For this review, take the finished solid that the model builds, in its own axes (mm). A direction names the side the tool comes from. Give positions to 0.01 mm unless a question says otherwise; leave off trailing zeros. Loops run counter-clockwise (first coordinate to the right, second up) from the corner with the lowest first, then second, coordinate; pieces in that order, holes last. Notation, with made-up numbers: (-11.5, -21.5) - (37.5, -21.5) arc R15 cw to (37.5, -8.5) - close; hole circle Ø9 at (2.5, 4). An arc over 180 degrees is marked (long way). Answer as CSV lines item,"result".
from build123d import *

# Parameters (mm, degrees)
F0_W     = 38.1
F0_H     = 12.7
F1_DEPTH = 25.4
F3_DEPTH = 12.7


with BuildPart() as f1:
    # F0 (on Front) → F1 (new body)
    with BuildSketch(Plane.XZ):
        with Locations((19.05, 6.35)):
            Rectangle(F0_W, F0_H)
    extrude(amount=F1_DEPTH)

    # F2 (on Front) → F3 (join)
    with BuildSketch(Plane.XZ):
        Polygon((0, 31.995658), (0, 12.945658), (0, 0), (38.1, 0), (38.1, 31.995658), (25.4, 31.995658), (25.4, 25.645658), (12.7, 25.645658), (12.7, 31.995658), align=None)
    extrude(amount=F3_DEPTH)


solid = f1.part
1) Consider section B-B on y = -7.75. Write out the cut boundary in (x, z).
From the geometry:
outline,"(0, 0) - (38.1, 0) - (38.1, 32) - (25.4, 32) - (25.4, 25.65) - (12.7, 25.65) - (12.7, 32) - (0, 32) - close"
2) Wall thickness on line 1 (Z direction, x = 16.5, y = -9.25); line 2 (Z direction, x = 20.5, y = -23); line 3 (Y direction, x = 24, z = 21.5): over which ranges is each line inside the solid? List them lowest first. Write a range as from..to.
From the geometry:
line 1,"z = 0..25.65"
line 2,"z = 0..12.7"
line 3,"y = -12.7..0"
3) Insertion check: P1, Ø14, axis at x = 26, y = -20, coming from the +Z side; P2, Ø4, axis at x = 16, y = -8.5, coming from the +Z side; P3, Ø5, axis at x = 18, z = 22.5, coming from the -Y side. Each pin has a flat end and moves straight along its axis. Give the tip position at first contact, or say it passes through.
From the geometry:
P1,"stops at z = 12.7"
P2,"stops at z = 25.65"
P3,"stops at y = -12.7"
4) Consider section C-C on x = 7. Write out the cut boundary in (y, z).
From the geometry:
outline,"(-25.4, 0) - (0, 0) - (0, 32) - (-12.7, 32) - (-12.7, 12.7) - (-25.4, 12.7) - close"
5) Consider section D-D on z = 14. Write out the cut boundary in (x, y), and give its area (3 significant figures).
From the geometry:
outline,"(0, -12.7) - (38.1, -12.7) - (38.1, 0) - (0, 0) - close"
area,"484 mm^2"
6) Draft analysis for pull direction X (two halves, no side actions). For faces 1 (the flat face through (19, -19, 12.7)), 2 (the flat face through (25.4, -6, 29)), 3 (the flat face through (0, -10, 13)), state which applies: pulls with the +X half, pulls with the -X half, needs draft (parallel to the pull), parting line crosses it, or undercut.
From the geometry:
face 1,"needs draft"
face 2,"undercut"
face 3,"pulls with the -X half"
7) Consider section A-A on z = 28. Write out the cut boundary in (x, y), and give its area (3 significant figures).
From the geometry:
outline,"(0, -12.7) - (12.7, -12.7) - (12.7, 0) - (0, 0) - close; (25.4, -12.7) - (38.1, -12.7) - (38.1, 0) - (25.4, 0) - close"
area,"323 mm^2"
8) Machinability: for faces 4 (the flat face through (19, 0, 16)), 5 (the flat face through (12.7, -6, 29)), 6 (the flat face through (19, -12.7, 22)), which of the approach directions +Z, -Z, +X, -X, +Y, -Y give a long, thin tool a straight path to every point of the face, cutting with its end or side? Answer none if there is none.
From the geometry:
face 4,"+Z, -Z, +X, -X, +Y"
face 5,"+Z, +Y, -Y"
face 6,"+Z, +X, -X, -Y"
